Model file for the job. Use its own axes, mm. A direction names the side the tool comes from. Coordinates: 2 decimals unless noted, no trailing zeros. Order: outer loops, then holes, each group sorted by start corner. A loop starts at its lowest first (then second) coordinate and runs counter-clockwise, first axis right, second up. Notation, with made-up numbers: (-9.5, 74.25) -> (41.5, 74.25) arc R25 cw to (41.5, 96.25) -> close; hole circle Ø6 at (72, -39). An arc over 180 degrees is marked (long way). Use CSV: the item, a comma, the result in double quotes. Start each with the question number.
(1) Pin check, flat tips, straight feed: pin 1 Ø2 at (y, z) = (3.5, 7.5) entering from -X; pin 2 Ø3 at (x, y) = (1, -4) entering from +Z; pin 3 Ø3.5 at (x, y) = (-0.5, -4) entering from +Z. Stop position of each tip, or through.
(2) Cut at B-B on z = 6.25. Write the cut outline in (x, y).
(3) Pull direction Y, two halves, no side cores. Call faces 4 (the flat face through (-3, 4.3, 8)), 5 (the cylindrical face through (3.72, -1.65, 8.84)), 6 (the cylindrical face through (0.05, -5.14, 6.05)): pulls with the +Y half, pulls with the -Y half, needs draft (parallel to the pull), parting line crosses it, or undercut.
(4) Probe L1, parallel to Z at x = 2.5, y = -4.75; L2, parallel to Z at x = 3, y = -3.5; L3, parallel to X at y = -2, z = 6.25. List the from-to ranges inside material, lowest first.
(5) Cut at A-A on y = 3.75. Write the cut outline in (x, z), plus the area to 3 significant figures.
(6) Tool access for faces 1 (the flat face through (1.5, -4, 3)), 2 (the flat face through (-3.9, 3, 8)), 3 (the cylindrical face through (-0.04, -4.34, 5.56)): list every direction of +Z, -Z, +X, -X, +Y, -Y with a clear straight run to the whole face (end or side of a thin tool).
```python
from build123d import *

# Parameters (mm, degrees)
PAD011_DEPTH      = 2
PAD011_DEPTH_BACK = 7.5
POCKET004_DEPTH   = 6.4
POCKET005_DEPTH   = 2.5
PAD013_DEPTH      = 0.45
PAD013_DEPTH_BACK = 0.45
FILLET023_R       = 0.5
FILLET025_R       = 0.2
FILLET024_R       = 0.2
FILLET020_R       = 0.5
SKETCH021_W       = 3
SKETCH021_H       = 1
PAD012_DEPTH      = 1
FILLET022_R       = 0.5
FILLET021_R       = 0.99


with BuildPart() as part:
    # Sketch019 (on DatumPlane) → Pad011 (new body, two sides)
    with BuildSketch(Plane.XY.offset(10)) as pad011_sk:
        with BuildLine():
            ThreePointArc((5.5, 1.920538), (0, 2.6), (-5.5, 1.920538))
            Line((-5.5, 1.920538), (-3.616372, -5.586761))
            ThreePointArc((3.616372, -5.586761), (0, -5.14), (-3.616372, -5.586761))
            Line((3.616372, -5.586761), (5.5, 1.920538))
        make_face()
    extrude(amount=PAD011_DEPTH)
    extrude(pad011_sk.sketch, amount=-PAD011_DEPTH_BACK)

    # Sketch017 (on Face5 of Pad011) → Pocket004 (cut)
    with BuildSketch(Plane(origin=(0, 0, 2.5), x_dir=(1, 0, 0), z_dir=(0, 0, -1))):
        with BuildLine():
            ThreePointArc((-4.515394, -1.283614), (0, -1.8), (4.515394, -1.283614))
            Line((3.020793, 4.673197), (4.515394, -1.283614))
            ThreePointArc((-3.020793, 4.673197), (0, 4.34), (3.020793, 4.673197))
            Line((-4.515394, -1.283614), (-3.020793, 4.673197))
        make_face()
    extrude(amount=-POCKET004_DEPTH, mode=Mode.SUBTRACT)

    # Sketch018 (on Face5 of Pocket004) → Pocket005 (cut)
    with BuildSketch(Plane.XY.offset(12)):
        with BuildLine():
            ThreePointArc((4.283186, -2.929138), (0, -2.4), (-4.283186, -2.929138))
            Line((-4.283186, -2.929138), (-3.616372, -5.586761))
            ThreePointArc((3.616372, -5.586761), (0, -5.14), (-3.616372, -5.586761))
            Line((4.283186, -2.929138), (3.616372, -5.586761))
        make_face()
    extrude(amount=-POCKET005_DEPTH, mode=Mode.SUBTRACT)

    # Sketch020 (on DatumPlane) → Pad013 (join, two sides)
    with BuildSketch(Plane.XY.offset(7.95)) as pad013_sk:
        Polygon((-3.9, 2.260952), (-3.9, 4.3), (-3, 4.3), (-2.1, 4.3), (-2.1, 2.502222), align=None)
        Polygon((2.1, 2.502222), (2.1, 4.3), (3, 4.3), (3.9, 4.3), (3.9, 2.260952), align=None)
    extrude(amount=PAD013_DEPTH)
    extrude(pad013_sk.sketch, amount=-PAD013_DEPTH_BACK)

    # Fillet023
    fillet023_edges = [part.edges().sort_by_distance(p)[0] for p in [
        (0, -2.4, 12),
        (4.891593, -0.5043, 12),
        (0, 2.6, 12),
        (-4.891593, -0.5043, 12),
        (4.283186, -2.929138, 10.75),
        (5.5, 1.920538, 7.25),
        (-5.5, 1.920538, 7.25),
        (-4.283186, -2.929138, 10.75),
    ]]
    fillet(fillet023_edges, radius=FILLET023_R)

    # Fillet025
    fillet025_edges = [part.edges().sort_by_distance(p)[0] for p in [
        (-3.616372, -5.586761, 6),
        (3.616372, -5.586761, 6),
        (-4.496657, -2.078339, 2.5),
        (4.496657, -2.078339, 2.5),
    ]]
    fillet(fillet025_edges, radius=FILLET025_R)

    # Fillet024
    fillet024_edges = [part.edges().sort_by_distance(p)[0] for p in [
        (0, -4.34, 8.9),
        (-3.768094, -1.694791, 8.9),
        (0, 1.8, 8.9),
        (3.768094, -1.694791, 8.9),
        (4.515394, 1.283614, 5.7),
        (3.020793, -4.673197, 5.7),
        (-3.020793, -4.673197, 5.7),
        (-4.515394, 1.283614, 5.7),
    ]]
    fillet(fillet024_edges, radius=FILLET024_R)

    # Fillet020
    fillet020_edges = [part.edges().sort_by_distance(p)[0] for p in [
        (-3.002424, 2.399675, 8.4),
        (-3.002424, 2.399675, 7.5),
        (3.002424, 2.399675, 7.5),
        (3.002424, 2.399675, 8.4),
    ]]
    fillet(fillet020_edges, radius=FILLET020_R)

    # Sketch021 (on Face21 of Fillet020) → Pad012 (join)
    with BuildSketch(Plane(origin=(0, 0, 2.5), x_dir=(1, 0, 0), z_dir=(0, 0, -1))):
        with Locations((0, 3.921408)):
            Rectangle(SKETCH021_W, SKETCH021_H)
    extrude(amount=-PAD012_DEPTH)

    # Fillet022
    fillet022_edges = [part.edges().sort_by_distance(p)[0] for p in [
        (0, -4.34, 3.5),
    ]]
    fillet(fillet022_edges, radius=FILLET022_R)

    # Fillet021
    fillet021_edges = [part.edges().sort_by_distance(p)[0] for p in [
        (0, -3.421408, 3.5),
    ]]
    fillet(fillet021_edges, radius=FILLET021_R)


solid = part.part
```
Outcome:
1,pin 1,"x = -3.9"
1,pin 2,"z = 9.5"
1,pin 3,"z = 11.86"
2,outline,"(-5.38, 1.43) -> (-3.66, -5.39) arc R0.2 ccw to (-3.42, -5.54) arc R14.86 cw to (3.42, -5.54) arc R0.2 ccw to (3.66, -5.39) -> (5.38, 1.43) arc R0.5 ccw to (5, 2.04) arc R22.6 ccw to (-5, 2.04) arc R0.5 ccw to start; hole (-4.47, 1.09) -> (-3.07, -4.49) arc R0.2 ccw to (-2.83, -4.63) arc R13.86 cw to (2.83, -4.63) arc R0.2 ccw to (3.07, -4.49) -> (4.47, 1.09) arc R0.2 ccw to (4.31, 1.33) arc R20 ccw to (-4.31, 1.33) arc R0.2 ccw to start"
3,face 4,"pulls with the +Y half"
3,face 5,"undercut"
3,face 6,"pulls with the -Y half"
4,L1,"2.5 to 9.5"
4,L2,"8.9 to 9.5"
4,L3,"-4.52 to -3.69, 3.69 to 4.52"
5,outline,"(-3.9, 7.5) -> (-2.1, 7.5) -> (-2.1, 8.4) -> (-3.9, 8.4) -> close; (2.1, 7.5) -> (3.9, 7.5) -> (3.9, 8.4) -> (2.1, 8.4) -> close"
5,area,"3.24 mm2"
6,face 1,"-Z"
6,face 2,"+Z, -Z, -X, +Y"
6,face 3,"none"
